```python
from build123d import *

# Parameters (mm, degrees)
SKETCH_1_W                  = 130
SKETCH_1_H                  = 100
EXTRUDE_1_DEPTH             = 2
FILLET_1_R                  = 5
SKETCH_2_R                  = 1.65
CUT_EXTRUDE_1_DEPTH         = 2
PATTERN_LINEAR_1_COUNT      = 2
PATTERN_LINEAR_1_PITCH      = 120
PATTERN_LINEAR_1_COUNT_DIR2 = 10
PATTERN_LINEAR_1_PITCH_DIR2 = 10
CUT_EXTRUDE_2_DEPTH         = 2


with BuildPart() as part:
    # 草图1 → 凸台-拉伸1 (new body)
    with BuildSketch(Plane.XY):
        with Locations((65, 50)):
            Rectangle(SKETCH_1_W, SKETCH_1_H)
    extrude(amount=EXTRUDE_1_DEPTH)

    # 圆角1
    fillet_1_edges = [part.edges().sort_by_distance(p)[0] for p in [
        (0, 100, 1),
        (130, 100, 1),
        (130, 0, 1),
        (0, 0, 1),
    ]]
    fillet(fillet_1_edges, radius=FILLET_1_R)

    # 草图2 → 切除-拉伸1 (cut)
    with BuildSketch(Plane.XY.offset(2)):
        with Locations((5, 95)):
            Circle(SKETCH_2_R)
    cut_extrude_1 = extrude(amount=-CUT_EXTRUDE_1_DEPTH, mode=Mode.SUBTRACT)

    # 阵列(线性)1: Cut-Extrude 1 2 × 10
    with Locations(*[(i * PATTERN_LINEAR_1_PITCH, -j * PATTERN_LINEAR_1_PITCH_DIR2, 0) for i in range(PATTERN_LINEAR_1_COUNT) for j in range(PATTERN_LINEAR_1_COUNT_DIR2) if (i, j) != (0, 0)]):
        add(cut_extrude_1, mode=Mode.SUBTRACT)

    # 草图3 → 切除-拉伸2 (cut)
    with BuildSketch(Plane.XY.offset(2)):
        with BuildLine():
            Line((37.866154951, 73.279191598), (90.557089201, 73.279191598))
            ThreePointArc((90.557089201, 73.279191598), (95.658146272, 78.380248669), (90.557089201, 83.48130574))
            Line((90.557089201, 83.48130574), (37.866154951, 83.48130574))
            ThreePointArc((37.866154951, 83.48130574), (32.76509788, 78.380248669), (37.866154951, 73.279191598))
        make_face()
        with BuildLine():
            ThreePointArc((90.557089201, 26.720808402), (95.658146272, 21.619751331), (90.557089201, 16.51869426))
            Line((90.557089201, 16.51869426), (37.866154951, 16.51869426))
            ThreePointArc((37.866154951, 16.51869426), (32.76509788, 21.619751331), (37.866154951, 26.720808402))
            Line((37.866154951, 26.720808402), (90.557089201, 26.720808402))
        make_face()
    extrude(amount=-CUT_EXTRUDE_2_DEPTH, mode=Mode.SUBTRACT)


solid = part.part
```
Source: CAD feature listing. Evaluate the final solid. Frame: model axes, mm. A direction names the side the tool comes from. Coordinates: 2 decimals unless noted, no trailing zeros. Loops run counter-clockwise (first coordinate to the right, second up) from the corner with the lowest first, then second, coordinate; pieces in that order, holes last. Notation, with made-up numbers: (25, 32) -> (84, 32) arc R27 cw to (84, 68) -> close; hole circle Ø10 at (75.5, 37). An arc over 180 degrees is marked (long way). One line per item, written item: value. Start each with the question number.
Q1. Section query C-C, the plane z = 0.85. Give the number of separate pieces and of enclosed holes in the cut face, and give its area (3 significant figures).
Q2. Section query A-A, the plane y = 45. Return the cut outline in (x, z).
Q3. Section query D-D, the plane y = 25. Return the cut outline in (x, z), and give its area (3 significant figures).
Q4. Mould query, pull axis X, two halves, no side actions, for faces 3 (the face through (126.574, 45.496, 1.014)), 4 (the face through (64, 51, 0)), 5 (the face through (1, 98, 1)). Classes: pulls with the +X half, pulls with the -X half, needs draft (parallel to the pull), parting line crosses it, or undercut.
Q5. Section query B-B, the plane x = 62. Return the cut outline in (y, z), and give its area (3 significant figures).
Q6. Set-up query: faces 1 (the face through (129, 98, 1)), 2 (the face through (95.657, 78.268, 1.014)). Return all of +Z, -Z, +X, -X, +Y, -Y with unobstructed straight access to the full face (end or side cutting, diameter ignored); none if empty.
Q7. Line query: line 1 along Y through (x, z) = (55, 0.25); line 2 along X through (y, z) = (65, 1.6); line 3 along X through (y, z) = (64, 1.6). Output: solid intervals per line, ascending.
Q8. Contact query for a flat-ended pin moving along its axis: P1, Ø3, axis at x = 125, y = 55, coming from the -Z side. Output: stop coordinate, or through.
Results:
1. separate pieces: 1
1. enclosed holes: 22
1. area: 11,600 mm^2
2. outline: (0, 0) -> (3.35, 0) -> (3.35, 2) -> (0, 2) -> close; (6.65, 0) -> (123.35, 0) -> (123.35, 2) -> (6.65, 2) -> close; (126.65, 0) -> (130, 0) -> (130, 2) -> (126.65, 2) -> close
3. outline: (0, 0) -> (3.35, 0) -> (3.35, 2) -> (0, 2) -> close; (6.65, 0) -> (34.05, 0) -> (34.05, 2) -> (6.65, 2) -> close; (94.38, 0) -> (123.35, 0) -> (123.35, 2) -> (94.38, 2) -> close; (126.65, 0) -> (130, 0) -> (130, 2) -> (126.65, 2) -> close
3. area: 126 mm^2
4. face 3: undercut
4. face 4: needs draft
4. face 5: pulls with the -X half
5. outline: (0, 0) -> (16.52, 0) -> (16.52, 2) -> (0, 2) -> close; (26.72, 0) -> (73.28, 0) -> (73.28, 2) -> (26.72, 2) -> close; (83.48, 0) -> (100, 0) -> (100, 2) -> (83.48, 2) -> close
5. area: 159 mm^2
6. face 1: +Z, -Z, +X, +Y
6. face 2: +Z, -Z
7. line 1: 0 to 16.52, 26.72 to 73.28, 83.48 to 100
7. line 2: 0 to 3.35, 6.65 to 123.35, 126.65 to 130
7. line 3: 0 to 3.69, 6.31 to 123.69, 126.31 to 130
8. P1: through
